Read the model definition and answer for the solid it produces. Units are mm, in the model's axes. Face numbers are marked on the shaded views. A direction names the side the tool comes from. Round coordinates to 2 decimals unless told otherwise and drop trailing zeros. Order: outer loops, then holes, each group sorted by start corner. A loop starts at its lowest first (then second) coordinate and runs counter-clockwise, first axis right, second up.
from build123d import *

# Parameters (mm, degrees)
F0_W      = 82.55
F0_H      = 34.798
F1_DEPTH  = 63.5
F2_W      = 31.75
F2_H      = 4.826
F3_DEPTH  = 63.501
F5_DEPTH  = 19.05
F7_DEPTH  = 82.551
F9_DEPTH  = 4.826
F10_R     = 6.35
F11_DEPTH = 15.749
F12_R     = 9.525
F13_DEPTH = 8.89


with BuildPart() as f1:
    # F0 (on Front) → F1 (new body)
    with BuildSketch(Plane.XZ):
        Rectangle(F0_W, F0_H)
    extrude(amount=F1_DEPTH)

    # F2 (on face) → F3 (cut, through all)
    with BuildSketch(Plane.XZ.offset(63.5)):
        with Locations((-25.4, -14.986)):
            Rectangle(F2_W, F2_H)
        with Locations((25.4, -14.986)):
            Rectangle(F2_W, F2_H)
    extrude(amount=-F3_DEPTH, mode=Mode.SUBTRACT)

    # F4 (on face) → F5 (cut)
    with BuildSketch(Plane.XY.offset(17.399)):
        Polygon((-1.676516, -23.876), (-34.925, -63.5), (41.275, -63.5), (41.275, 0), (-1.676516, 0), align=None)
    extrude(amount=-F5_DEPTH, mode=Mode.SUBTRACT)

    # F6 (on face) → F7 (cut, through all)
    with BuildSketch(Plane(origin=(-41.275, 0, 0), x_dir=(0, -1, 0), z_dir=(-1, 0, 0))):
        Polygon((0, 17.399), (0, 3.614185), (23.876, 17.399), align=None)
    extrude(amount=-F7_DEPTH, mode=Mode.SUBTRACT)

    # F8 (on face) → F9 (cut)
    with BuildSketch(Plane.XY.offset(-1.651)):
        Polygon((15.875, -63.5), (41.275, -63.5), (41.275, -33.229459), align=None)
    extrude(amount=-F9_DEPTH, mode=Mode.SUBTRACT)

    # F10 (on face) → F11 (cut, through all)
    with BuildSketch(Plane.XY.offset(-1.651)):
        with Locations((0, -44.45)):
            Circle(F10_R)
    extrude(amount=-F11_DEPTH, mode=Mode.SUBTRACT)

    # F12 (on face) → F13 (cut)
    with BuildSketch(Plane.XY.offset(-1.651)):
        with Locations((0, -44.45)):
            Circle(F12_R)
    extrude(amount=-F13_DEPTH, mode=Mode.SUBTRACT)


solid = f1.part
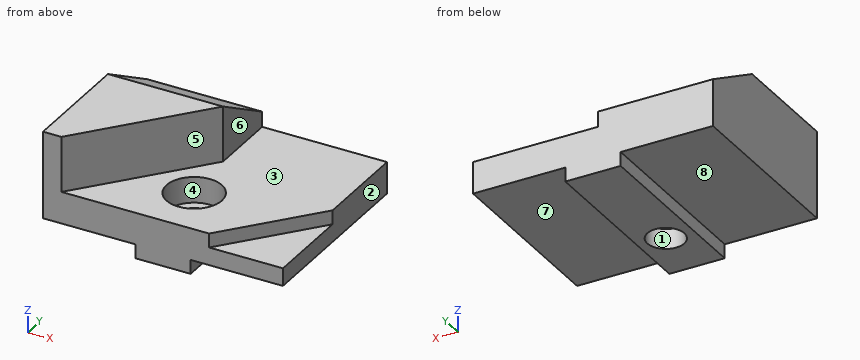
Q1. For a pull along X with two mould halves and no side action, classify the marked faces 1, 2, 3 and 4 as released by +X, released by -X, zero draft, split by the parting line, or undercut.
Outcome:
face 1: undercut
face 2: released by +X
face 3: zero draft
face 4: undercut
Q2. For the marked faces 5, 6, 7 and 8, determine the directions among +Z, -Z, +X, -X, +Y, -Y from which every point of the face is accessible in a straight line to the end or side of a thin tool.
Outcome:
face 5: +Z, +X, -Y
face 6: +Z, +X, +Y, -Y
face 7: -Z, +X, +Y, -Y
face 8: -Z, -X, +Y, -Y
Q3. A cutting plane is placed at A-A, the plane x = 0. Give the vertices of the cut face in (y, z) (3 decimals).
Outcome:
outline: (-63.5, -17.399) - (-50.8, -17.399) - (-50.8, -10.541) - (-53.975, -10.541) - (-53.975, -1.651) - (-63.5, -1.651) - close; (-38.1, -17.399) - (0, -17.399) - (0, -1.651) - (-34.925, -1.651) - (-34.925, -10.541) - (-38.1, -10.541) - close
Q4. A cutting plane is placed at C-C, the plane z = -8.5. Give the vertices of the cut face in (x, y) (3 decimals).
Outcome:
outline: (-41.275, -63.5) - (41.275, -63.5) - (41.275, 0) - (-41.275, 0) - close; hole circle Ø19.05 at (0, -44.45)
Q5. A cutting plane is placed at D-D, the plane x = -17. Give the vertices of the cut face in (y, z).
Outcome:
outline: (-63.5, -12.57) - (0, -12.57) - (0, 3.61) - (-23.88, 17.4) - (-42.14, 17.4) - (-42.14, -1.65) - (-63.5, -1.65) - close
Q6. Straight lines are drawn through the part: probe 1 along X at (y, z) = (-44, -12) (3 decimals); probe 2 along Y at (x, z) = (0, -12.5); probe 3 along Y at (x, z) = (0, -7) (3 decimals). For each, find the intervals that lie inside material, in ascending order.
Outcome:
probe 1: x = -41.275 to -6.334, 6.334 to 41.275
probe 2: y = -63.5 to -50.8, -38.1 to 0
probe 3: y = -63.5 to -53.975, -34.925 to 0
Q7. A cutting plane is placed at B-B, the plane y = -42. Give the vertices of the cut face in (x, z) (3 decimals), plus the area to 3 significant figures.
Outcome:
outline: (-41.275, -12.573) - (-9.525, -12.573) - (-9.525, -17.399) - (-5.858, -17.399) - (-5.858, -10.541) - (-9.205, -10.541) - (-9.205, -1.651) - (-16.884, -1.651) - (-16.884, 17.399) - (-41.275, 17.399) - close; (5.858, -17.399) - (9.525, -17.399) - (9.525, -12.573) - (41.275, -12.573) - (41.275, -6.477) - (33.916, -6.477) - (33.916, -1.651) - (9.205, -1.651) - (9.205, -10.541) - (5.858, -10.541) - close
area: 1,180 mm2
Q8. Flat-ended cylindrical pins translate along their axes: pin 1 (10 mm diameter, centred on x = -9, z = 5.5, fed in from -Y); pin 2 (1.4 mm diameter, centred on y = -21.5, z = -16, fed in from -X) (3 decimals); pin 3 (1 mm diameter, centred on x = -14, z = -2.5, fed in from +Y); pin 4 (8 mm diameter, centred on x = 19, y = -16.5, fed in from -Z). Find the tip coordinate at first contact, or state that the pin passes through.
Outcome:
pin 1: stops at y = -38.56
pin 2: stops at x = -9.525
pin 3: stops at y = 0
pin 4: stops at z = -12.57
